Check sheet for the modelled part. Datum: model origin and axes. Units: mm. A direction names the side the tool comes from. Give positions to 0.01 mm unless a question says otherwise; leave off trailing zeros. Write each loop counter-clockwise with the first axis right and the second up, starting at its lowest first coordinate (ties: lowest second). Pieces come first, ordered by that corner, then holes. Notation, with made-up numbers: (17.5, 23) - (49.5, 23) arc R21 ccw to (49.5, 38) - close; hole circle Ø1 at (14, -34). An arc over 180 degrees is marked (long way). Return JSON: item names as keys, results as strings. Group by question number.
```python
from build123d import *

# Parameters (mm, degrees)
BOSS_EXTRUDE1_DEPTH = 44.45
BOSS_EXTRUDE2_DEPTH = 57.15
SKETCH5_R           = 9.525
CUT_EXTRUDE1_DEPTH  = 6.35
SKETCH6_R           = 9.525
CUT_EXTRUDE2_DEPTH  = 6.35
SKETCH7_R           = 4.7625
CUT_EXTRUDE3_DEPTH  = 12.7


with BuildPart() as part:
    # Sketch1 → Boss-Extrude1 (new body)
    with BuildSketch(Plane.XY):
        Polygon((0, 0), (0, 50.862487244), (57.248927697, 50.862487244), (57.248927697, 24.680871047), (88.998927697, 6.35), (88.998927697, 0), align=None)
    extrude(amount=BOSS_EXTRUDE1_DEPTH)

    # Sketch2 → Boss-Extrude2 (add)
    with BuildSketch(Plane(origin=(57.248927697, 0, 0), x_dir=(0, 0, -1), z_dir=(1, 0, 0))):
        Polygon((-44.45, 50.862487244), (-80.305183767, 30.161487244), (-73.955183767, 19.162964616), (-44.45, 36.197790407), align=None)
    extrude(amount=-BOSS_EXTRUDE2_DEPTH)

    # Sketch5 → Cut-Extrude1 (cut)
    with BuildSketch(Plane(origin=(0, 57.394280032, 33.136603026), x_dir=(1, 0, 0), z_dir=(0, 0.866025404, 0.5))):
        with Locations((28.800927697, -35.415585576)):
            Circle(SKETCH5_R)
    extrude(amount=-CUT_EXTRUDE1_DEPTH, mode=Mode.SUBTRACT)

    # Sketch6 → Cut-Extrude2 (cut)
    with BuildSketch(Plane(origin=(24.999362581, 43.300166148, 0), x_dir=(0.866025404, -0.5, 0), z_dir=(0.5, 0.866025404, 0))):
        with Locations((54.850332296, -22.098)):
            Circle(SKETCH6_R)
    extrude(amount=-CUT_EXTRUDE2_DEPTH, mode=Mode.SUBTRACT)

    # Sketch7 → Cut-Extrude3 (cut)
    with BuildSketch(Plane(origin=(0, 50.862487244, 0), x_dir=(1, 0, 0), z_dir=(0, 1, 0))):
        with Locations((15.846927697, -12.7)):
            Circle(SKETCH7_R)
        with Locations((15.846927697, -31.75)):
            Circle(SKETCH7_R)
        with Locations((41.246927697, -31.75)):
            Circle(SKETCH7_R)
        with Locations((41.246927697, -12.7)):
            Circle(SKETCH7_R)
    extrude(amount=-CUT_EXTRUDE3_DEPTH, mode=Mode.SUBTRACT)


solid = part.part
```
Item 1: Mould release check, pull along X, two halves, no side actions. Record for faces 4 (the face through (37.886, 38.406, 59.764)), 5 (the face through (57.249, 39, 32)), 6 (the face through (45, 0, 22)): +X half, -X half, draft (parallel to the pull), parting line (faces both ways), or undercut.
Item 2: Section check C-C on z = 38.5. Record the cut outline in (x, y), plus the area to 3 significant figures.
Item 3: Material ranges on line 1 along X through (y, z) = (43.75, 31.75); line 2 along X through (y, z) = (49, 16.5); line 3 along Z through (x, y) = (47.5, 3), recorded low to high. Write a range as from..to.
Item 4: Section check A-A on z = 14.5. Record the cut outline in (x, y).
Item 5: Section check B-B on x = 17. Record the cut outline in (y, z).
Item 6: Access from +Z, -Z, +X, -X, +Y, -Y to the whole of each face (thin tool, end or side, straight path). Record for faces 1 (the face through (0.099, 35, 63)), 2 (the face through (69.211, 10.442, 21.965)), 3 (the face through (45.79, 44.6, 30.32)).
Item 7: Section check D-D on x = 29. Record the cut outline in (y, z), plus the area to 3 significant figures.
Item 8: Depth check by flat-ended pin: pin 1 (5 mm diameter, centred on x = 49.5, y = 21.5, fed in from -Z); pin 2 (6 mm diameter, centred on y = 38.5, z = 28.5, fed in from +X); pin 3 (7.5 mm diameter, centred on x = 41.25, z = 31.75, fed in from +Y); pin 4 (16 mm diameter, centred on y = 28, z = 22, fed in from +X). Enter the tip coordinate at first touch or a pass-through.
Reply:
{
 "1": {"face 4": "undercut", "face 5": "+X half", "face 6": "draft"},
 "2": {"outline": "(0, 0) - (89, 0) - (89, 6.35) - (57.25, 24.68) - (57.25, 50.86) - (0, 50.86) - close", "area": "3,400 mm²"},
 "3": {"line 1": "0..11.08, 20.61..36.48, 46.01..57.25", "line 2": "0..12.98, 18.72..38.38, 44.12..57.25", "line 3": "0..44.45"},
 "4": {"outline": "(0, 0) - (89, 0) - (89, 6.35) - (77.48, 13) - (74.3, 7.5) - (64.35, 13.25) - (67.53, 18.75) - (57.25, 24.68) - (57.25, 50.86) - (45.66, 50.86) - (45.66, 38.16) - (36.84, 38.16) - (36.84, 50.86) - (20.26, 50.86) - (20.26, 38.16) - (11.44, 38.16) - (11.44, 50.86) - (0, 50.86) - close"},
 "5": {"outline": "(0, 0) - (50.86, 0) - (50.86, 8.08) - (38.16, 8.08) - (38.16, 17.32) - (50.86, 17.32) - (50.86, 27.13) - (38.16, 27.13) - (38.16, 36.37) - (50.86, 36.37) - (50.86, 44.45) - (30.16, 80.31) - (19.16, 73.96) - (36.2, 44.45) - (0, 44.45) - close"},
 "6": {"face 1": "+Z, -X, +Y, -Y", "face 2": "none", "face 3": "+Y"},
 "7": {"outline": "(0, 0) - (50.86, 0) - (50.86, 44.45) - (44.45, 55.56) - (38.95, 52.39) - (29.43, 68.88) - (34.93, 72.05) - (30.16, 80.31) - (19.16, 73.96) - (36.2, 44.45) - (0, 44.45) - close", "area": "2,620 mm²"},
 "8": {"pin 1": "z = 0", "pin 2": "x = 57.25", "pin 3": "y = 38.16", "pin 4": "x = 64.59"}
}
